Work out the finished part from the listing and answer in its coordinate system (mm). Face numbers are marked on the shaded views. A direction names the side the tool comes from. Give positions to 0.01 mm unless a question says otherwise; leave off trailing zeros. Loops run counter-clockwise (first coordinate to the right, second up) from the corner with the lowest first, then second, coordinate; pieces in that order, holes last. Notation, with made-up numbers: (26.25, 76.5) - (46.25, 76.5) arc R29 ccw to (46.25, 97.5) - close; hole circle Ø8 at (-40, 60). An arc over 180 degrees is marked (long way). One line per question, with ' | ' between items. Start each with the question number.
1. Each of these flat-tipped pins is pushed along its axis until it touches: pin 1 (24 mm diameter, centred on x = 12, y = 123, fed in from +Z); pin 2 (8 mm diameter, centred on x = 8, y = 118, fed in from -Z). Where does it stop, or does it pass through?
2. Section B-B (x = -17.5) is taken. Determine the outline of the cut face in (y, z).
3. Find the intervals of material crossed by line 1 (Y direction, x = 16, z = -24); line 2 (Z direction, x = -21, y = 140), in increasing order.
4. Which of the six approach directions +Z, -Z, +X, -X, +Y, -Y give full straight-line access (tool end or side, diameter ignored) to the marked faces 1, 2 and 3?
5. Section A-A (z = 17) is taken. Determine the outline of the cut face in (x, y).
6. For a pull along Y with two mould halves and no side action, classify the marked faces 4, 5, 6 and 7 as released by +Y, released by -Y, zero draft, split by the parting line, or undercut.
7. Section C-C (y = 171) is taken. Determine the outline of the cut face in (x, z), plus the area to 3 significant figures.
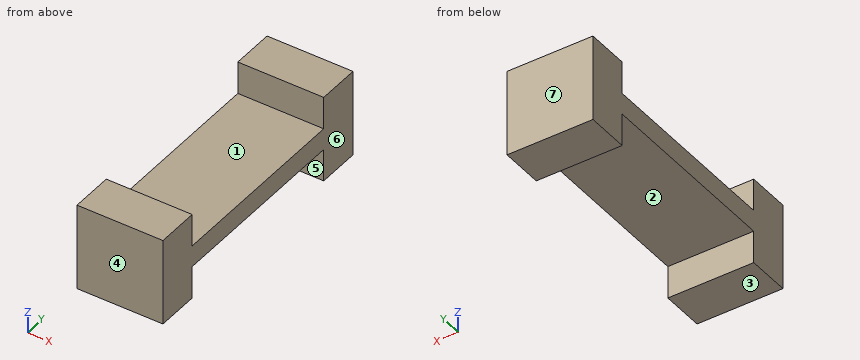
from build123d import *

# Parameters (mm, degrees)
SKETCH1_W           = 79.968077757
SKETCH1_H           = 80.704842411
BOSS_EXTRUDE1_DEPTH = 130
SKETCH2_W           = 30.352421206
SKETCH2_H           = 320
SKETCH2_W_2         = 30.352421205
CUT_EXTRUDE1_DEPTH  = 80
MIRROR3_START       = -31.568063376
MIRROR3_DEPTH       = 79.968077757


# Read off the part's stored shape, not the designer's step: Mirror3
with BuildPart() as part:
    # Sketch1 → Boss-Extrude1 (new body)
    with BuildSketch(Plane(origin=(0, 0, 0), x_dir=(1, 0, 0), z_dir=(0, 1, 0))):
        with Locations((8.415975503, -0.026706735)):
            Rectangle(SKETCH1_W, SKETCH1_H)
    extrude(amount=BOSS_EXTRUDE1_DEPTH)

    # Sketch2 → Cut-Extrude1 (cut)
    with BuildSketch(Plane(origin=(48.400014381, 0, 0), x_dir=(0, 0, -1), z_dir=(1, 0, 0))):
        with Locations((-25.202917338, 200)):
            Rectangle(SKETCH2_W, SKETCH2_H)
        with Locations((25.149503868, 200)):
            Rectangle(SKETCH2_W_2, SKETCH2_H)
    extrude(amount=-CUT_EXTRUDE1_DEPTH, mode=Mode.SUBTRACT)

    # Mirror3 outline → Mirror3 (add)
    with BuildSketch(Plane.YZ.offset(MIRROR3_START)):
        Polygon((220, -40.32571447), (260, -40.32571447), (260, 40.379127941), (220, 40.379127941), (220, 10.026706735), (130, 10.026706735), (130, -9.973293265), (220, -9.973293265), align=None)
    extrude(amount=MIRROR3_DEPTH)


solid = part.part
Conclusion:
1) pin 1: z = 10.03 | pin 2: z = -9.97
2) outline: (0, -40.33) - (40, -40.33) - (40, -9.97) - (220, -9.97) - (220, -40.33) - (260, -40.33) - (260, 40.38) - (220, 40.38) - (220, 10.03) - (40, 10.03) - (40, 40.38) - (0, 40.38) - close
3) line 1: 0 to 40, 220 to 260 | line 2: -9.97 to 10.03
4) face 1: +Z, +X, -X | face 2: -Z, +X, -X | face 3: -Z, +X, -X, +Y, -Y
5) outline: (-31.57, 0) - (48.4, 0) - (48.4, 40) - (-31.57, 40) - close; (-31.57, 220) - (48.4, 220) - (48.4, 260) - (-31.57, 260) - close
6) face 4: released by -Y | face 5: undercut | face 6: zero draft | face 7: released by +Y
7) outline: (-31.57, -9.97) - (48.4, -9.97) - (48.4, 10.03) - (-31.57, 10.03) - close | area: 1,600 mm²
